from build123d import *

# Parameters (mm, degrees)
CYLINDER098_R     = 1.5
CYLINDER098_DEPTH = 14
CYLINDER097_R     = 12
CYLINDER097_DEPTH = 33
CYLINDER099_R     = 1.5
CYLINDER099_DEPTH = 14
BOX017_W          = 47
BOX017_H          = 10
BOX017_DEPTH      = 5
CYLINDER096_R     = 17
CYLINDER096_DEPTH = 5


with BuildPart() as obj1:
    # Cylinder098 → Cylinder098 (new body)
    with BuildSketch(Plane(origin=(53.66, 148, -15), x_dir=(1, 0, 0), z_dir=(0, 0, 1))):
        Circle(CYLINDER098_R)
    extrude(amount=CYLINDER098_DEPTH)


with BuildPart() as obj2:
    # Cylinder097 → Cylinder097 (new body)
    with BuildSketch(Plane(origin=(73.66, 148, -10), x_dir=(1, 0, 0), z_dir=(0, 0, 1))):
        Circle(CYLINDER097_R)
    extrude(amount=CYLINDER097_DEPTH)


with BuildPart() as fusion041:
    # Cylinder099 → Cylinder099 (new body)
    with BuildSketch(Plane(origin=(93.66, 148, -14), x_dir=(1, 0, 0), z_dir=(0, 0, 1))):
        Circle(CYLINDER099_R)
    extrude(amount=CYLINDER099_DEPTH)

    # Fusion041: union obj1, obj2
    add(obj1.part)
    add(obj2.part)


with BuildPart() as obj3:
    # Box017 → Box017 (new body)
    with BuildSketch(Plane(origin=(50, 143, -10), x_dir=(1, 0, 0), z_dir=(0, 0, 1))):
        with Locations((23.5, 5)):
            Rectangle(BOX017_W, BOX017_H)
    extrude(amount=BOX017_DEPTH)


with BuildPart() as obj4:
    # Cylinder096 → Cylinder096 (new body)
    with BuildSketch(Plane(origin=(73.66, 148, -10), x_dir=(1, 0, 0), z_dir=(0, 0, 1))):
        Circle(CYLINDER096_R)
    extrude(amount=CYLINDER096_DEPTH)

    # Fusion042: union obj3
    add(obj3.part)

    # Cut011: cut Fusion041
    add(fusion041.part, mode=Mode.SUBTRACT)


with BuildPart() as obj4_1:
    # Cut011 placement: moved
    add(obj4.part.moved(Location((0, 0, -3))))


solid = obj4_1.part
The listing builds one solid part. Answer for the finished solid, in the listing's coordinates (mm). A direction names the side the tool comes from. Round coordinates to 2 decimals unless told otherwise and drop trailing zeros. Loops run counter-clockwise (first coordinate to the right, second up) from the corner with the lowest first, then second, coordinate; pieces in that order, holes last. Notation, with made-up numbers: M 69,24.5 L 83,24.5 A12 ccw 83,38.5 Z; hole C 59,76.5 d2. An arc over 180 degrees is marked long. Return JSON: item names as keys, results as strings.
Q1. Find section D-D, the plane y = 140.5. Determine the outline of the cut face in (x, z).
Results list:
{"outline": "M 58.4,-13 L 64.29,-13 L 64.29,-8 L 58.4,-8 Z; M 83.03,-13 L 88.92,-13 L 88.92,-8 L 83.03,-8 Z"}
Q2. Find section A-A, the plane x = 73.66. Determine the outline of the cut face in (y, z), plus the area to 3 significant figures.
Results list:
{"outline": "M 131,-13 L 136,-13 L 136,-8 L 131,-8 Z; M 160,-13 L 165,-13 L 165,-8 L 160,-8 Z", "area": "50.0 mm2"}
Q3. Each of these flat-tipped pins is pushed along its axis until it touches: pin 1 Ø14.5 at (x, y) = (73.66, 148) entering from -Z; pin 2 Ø1.5 at (y, z) = (154, -9.5) entering from +X; pin 3 Ø1.5 at (x, z) = (93, -11.5) entering from +Y; pin 4 Ø1.5 at (x, z) = (92, -10.5) entering from -Y. Where does it stop, or does it pass through?
Results list:
{"pin 1": "passes through", "pin 2": "stops at x = 89.83", "pin 3": "stops at y = 153", "pin 4": "stops at y = 143"}
Q4. Which of the six approach directions +Z, -Z, +X, -X, +Y, -Y give full straight-line access (tool end or side, diameter ignored) to faces 1 (the face through (54, 153, -11)), 2 (the face through (93, 153, -11)), 3 (the face through (93, 143, -11)), 4 (the face through (54, 143, -11)), 5 (the face through (92.55, 149.01, -10.54))?
Results list:
{"face 1": "+Z, -Z, -X, +Y", "face 2": "+Z, -Z, +X, +Y", "face 3": "+Z, -Z, +X, -Y", "face 4": "+Z, -Z, -X, -Y", "face 5": "+Z, -Z"}
Q5. Find the intervals of material crossed by line 1 along X through (y, z) = (148, -10.1); line 2 along Y through (x, z) = (53.66, -9.85); line 3 along Y through (x, z) = (74, -11.3), in increasing order. Write a range as from..to.
Results list:
{"line 1": "x = 50..52.16, 55.16..61.66, 85.66..92.16, 95.16..97", "line 2": "y = 143..146.5, 149.5..153", "line 3": "y = 131..136, 160..165"}
Q6. Find section B-B, the plane y = 148. Determine the outline of the cut face in (x, z), plus the area to 3 significant figures.
Results list:
{"outline": "M 50,-13 L 52.16,-13 L 52.16,-8 L 50,-8 Z; M 55.16,-13 L 61.66,-13 L 61.66,-8 L 55.16,-8 Z; M 85.66,-13 L 92.16,-13 L 92.16,-8 L 85.66,-8 Z; M 95.16,-13 L 97,-13 L 97,-8 L 95.16,-8 Z", "area": "85.0 mm2"}
Q7. Find section C-C, the plane z = -9.2. Determine the outline of the cut face in (x, y).
Results list:
{"outline": "M 50,143 L 57.41,143 A17 ccw 89.91,143 L 97,143 L 97,153 L 89.91,153 A17 ccw 57.41,153 L 50,153 Z; hole C 53.66,148 d3; hole C 73.66,148 d24; hole C 93.66,148 d3"}
Q8. The mould has two halves that part along X. Classify faces 6 (the face through (63, 142, -13)), 7 (the face through (54.466, 149.265, -10.535)), 8 (the face through (73.963, 164.997, -10.535)), 9 (the face through (50, 148, -11)): released by +X, released by -X, zero draft, split by the parting line, or undercut.
Results list:
{"face 6": "zero draft", "face 7": "undercut", "face 8": "split by the parting line", "face 9": "released by -X"}
